from build123d import *

# Parameters (mm, degrees)
SKETCH_1_R          = 90
EXTRUDE_1_DEPTH     = 20
SKETCH_2_R          = 90
EXTRUDE_2_DEPTH     = 20
SKETCH_3_R          = 68
CUT_EXTRUDE_1_DEPTH = 8
SKETCH_4_R          = 68
CUT_EXTRUDE_2_DEPTH = 8
SKETCH_5_R          = 75
SKETCH_7_R          = 51
SKETCH_8_R          = 75
SKETCH_9_R          = 51
SKETCH_11_W         = 21.388157758
SKETCH_11_H         = 3.979192142


with BuildPart() as part:
    # Sketch 1 → Extrude 1 (new body)
    with BuildSketch(Plane.XY):
        Circle(SKETCH_1_R)
    extrude(amount=EXTRUDE_1_DEPTH)

    # Sketch 4 → Cut-Extrude 2 (cut)
    with BuildSketch(Plane.XY.offset(20)):
        with Locations(Location((0, 0, 0), (0, 0, 180))):
            Circle(SKETCH_4_R)
    extrude(amount=-CUT_EXTRUDE_2_DEPTH, mode=Mode.SUBTRACT)

    # Sketch 8 → Loft 2 section 0
    with BuildSketch(Plane(origin=(0, 0, 0), x_dir=(-1, 0, 0), z_dir=(0, 0, -1))):
        Circle(SKETCH_8_R)
    # Sketch 9 → Loft 2 section 1
    with BuildSketch(Plane(origin=(0, 0, -5), x_dir=(-1, 0, 0), z_dir=(0, 0, -1))):
        Circle(SKETCH_9_R)
    loft()



with BuildPart() as body_2:
    # Sketch 2 → Extrude 2 (new body)
    with BuildSketch(Plane.XY.offset(300)):
        Circle(SKETCH_2_R)
    extrude(amount=EXTRUDE_2_DEPTH)

    # Sketch 3 → Cut-Extrude 1 (cut)
    with BuildSketch(Plane(origin=(0, 0, 300), x_dir=(-1, 0, 0), z_dir=(0, 0, -1))):
        Circle(SKETCH_3_R)
    extrude(amount=-CUT_EXTRUDE_1_DEPTH, mode=Mode.SUBTRACT)

    # Sketch 5 → Loft 1 section 0
    with BuildSketch(Plane.XY.offset(320)):
        Circle(SKETCH_5_R)
    # Sketch 7 → Loft 1 section 1
    with BuildSketch(Plane.XY.offset(325)):
        Circle(SKETCH_7_R)
    loft()


with BuildPart() as part_1:
    add(part.part)

    add(body_2.part)  # Sweep 1 merges body 2
    # Sweep 1: sweep along a path in Sketch 14
    with BuildLine(Plane(origin=(0, 0, 0), x_dir=(0, 0, -1), z_dir=(1, 0, 0))) as sweep_1_path:
        ThreePointArc((-5.541455061, -14.409759427), (-160.373186446, 291.522166595), (-315.20491783, -14.409759427))
    # Sketch 11 → Sweep 1 (sweep)
    with BuildSketch(Plane.XY.offset(325)):
        Rectangle(SKETCH_11_W, SKETCH_11_H)
    sweep(path=sweep_1_path.line)


solid = part_1.part
Model file for the job. Use its own axes, mm. A direction names the side the tool comes from. Round coordinates to 2 decimals unless told otherwise and drop trailing zeros. Loops run counter-clockwise (first coordinate to the right, second up) from the corner with the lowest first, then second, coordinate; pieces in that order, holes last.
1. Band-saw the part on A-A, the plane y = 251.5. List the corners of the cut face in (x, z).
Check values:
outline: (-10.69, 41.06) - (10.69, 41.06) - (10.69, 44.42) - (-10.69, 44.42) - close; (-10.69, 276.32) - (10.69, 276.32) - (10.69, 279.69) - (-10.69, 279.69) - close
2. Band-saw the part on B-B, the plane x = 0. List the corners of the cut face in (y, z) (3 decimals), and give its area (3 significant figures).
Check values:
outline: (-90, 0) - (-75, 0) - (-51, -5) - (-0.767, -5) arc R193.331 ccw (long way) to (-1.99, 325) - (-51, 325) - (-75, 320) - (-90, 320) - (-90, 300) - (-68, 300) - (-68, 308) - (68, 308) - (68, 300) - (90, 300) - (90, 320) - (75, 320) - (51, 325) - (1.99, 325) arc R191.275 cw (long way) to (3.262, -5) - (51, -5) - (75, 0) - (90, 0) - (90, 20) - (68, 20) - (68, 12) - (-68, 12) - (-68, 20) - (-90, 20) - close
area: 7,950 mm2
3. Mould opens along X. For faces 1 (the flat face through (1, -1, 12)), 2 (the flat face through (-20, 74, 0)), 3 (the flat face through (10.694, 287, 203)), 4 (the cylindrical face through (8.85, -67.42, 16.06)) say: +X half, -X half, draft (parallel to the pull), parting line (faces both ways), or undercut.
Check values:
face 1: undercut
face 2: draft
face 3: +X half
face 4: undercut
4. Drop flat-ended pins along their axis: P1, Ø12, axis at x = 46, y = -50.5, coming from the +Z side; P2, Ø4, axis at x = 7, y = 247, coming from the +Z side. Give the stop position or say it passes through.
Check values:
P1: stops at z = 322.64
P2: stops at z = 287.54
5. Band-saw the part on D-D, the plane z = 35. List the corners of the cut face in (x, y), and give its area (3 significant figures).
Check values:
outline: (-10.69, 243.83) - (10.69, 243.83) - (10.69, 246.54) - (-10.69, 246.54) - close
area: 58.0 mm2
6. Tool access for faces 5 (the flat face through (1, 1, 308)), 6 (the cylindrical face through (0.15, 292.642, 155.354)): list every direction of +Z, -Z, +X, -X, +Y, -Y with a clear straight run to the whole face (end or side of a thin tool).
Check values:
face 5: none
face 6: +X, -X
7. Wall check: probe 1 along Z at (x, y) = (-42.5, -70.5); probe 2 along Z at (x, y) = (-3, 97); probe 3 along Y at (x, z) = (0, 306.5). Give the ranges that are in metal, low to high.
Check values:
probe 1: z = 0 to 20, 300 to 320
probe 2: z = -32.94 to -30.89, 351.63 to 353.69
probe 3: y = -90 to -68, 68 to 90, 222.8 to 225.96
